Here's how the part is built. I have some questions about the finished solid (model axes, mm). A direction names the side the tool comes from. Coordinates: 2 decimals unless noted, no trailing zeros. Order: outer loops, then holes, each group sorted by start corner. A loop starts at its lowest first (then second) coordinate and runs counter-clockwise, first axis right, second up. Notation, with made-up numbers: M 62.5,10.5 L 77.5,10.5 A36 ccw 77.5,46.5 Z; hole C 52.25,15.5 d4. An arc over 180 degrees is marked long. One line per question, with ' | ' between items. Start each with the question number.
```python
from build123d import *

# Parameters (mm, degrees)
MAIN_5_W                = 20
MAIN_5_H                = 12.7
BOSS_EXTRUDE2_DEPTH     = 6.35
CUT_EXTRUDE1_DEPTH      = 300.179502974
CUT_EXTRUDE1_DEPTH_BACK = 300.179502974
SKETCH1_W               = 12.7
SKETCH1_H               = 20
M8_CLEARANCE_HOLE2_D    = 9
CUT_EXTRUDE2_DEPTH      = 300.179502974
CUT_EXTRUDE2_DEPTH_BACK = 300.179502974
SKETCH6_R               = 4
SKETCH6_R_2             = 3.175
SKETCH6_R_3             = 1.25
CUT_EXTRUDE3_DEPTH      = 300.179502974
CUT_EXTRUDE3_DEPTH_BACK = 300.179502974
SKETCH7_R               = 25
F_6_0MM_DOWEL_HOLE2_D   = 6


with BuildPart() as part:
    # MAIN<5> → Boss-Extrude2 (new, symmetric)
    with BuildSketch(Plane(origin=(0, 0, 0), x_dir=(1, 0, 0), z_dir=(0, 1, 0))):
        Polygon((-271.75, 92.5), (-271.75, 79.8), (-284.45, 79.8), (-284.45, 59.8), (-271.75, 59.8), (-271.75, 4), (-266.45, 4), (-266.45, 6.5), (-259.45, 6.5), (-259.45, 4), (-256.45, 4), (-256.45, -4), (-259.45, -4), (-259.45, -6.5), (-266.45, -6.5), (-266.45, -4), (-271.75, -4), (-271.75, -59.8), (-284.45, -59.8), (-284.45, -79.8), (-271.75, -79.8), (-271.75, -92.5), (271.75, -92.5), (271.75, -79.8), (284.45, -79.8), (284.45, -59.8), (271.75, -59.8), (271.75, -4), (266.45, -4), (266.45, -6.5), (259.45, -6.5), (259.45, -4), (256.45, -4), (256.45, 4), (259.45, 4), (259.45, 6.5), (266.45, 6.5), (266.45, 4), (271.75, 4), (271.75, 59.8), (284.45, 59.8), (284.45, 79.8), (271.75, 79.8), (271.75, 92.5), align=None)
        with Locations((-157.7, 0)):
            Rectangle(MAIN_5_W, MAIN_5_H, mode=Mode.SUBTRACT)
        with Locations((-107.7, 0)):
            Rectangle(MAIN_5_W, MAIN_5_H, mode=Mode.SUBTRACT)
        with Locations((107.7, 0)):
            Rectangle(MAIN_5_W, MAIN_5_H, mode=Mode.SUBTRACT)
        with Locations((157.7, 0)):
            Rectangle(MAIN_5_W, MAIN_5_H, mode=Mode.SUBTRACT)
    extrude(amount=BOSS_EXTRUDE2_DEPTH, both=True)

    # Sketch1 → Cut-Extrude1 (cut, two sides: drawn at the far end of the back side and taken through both)
    with BuildSketch(Plane(origin=(0, 0, 0), x_dir=(1, 0, 0), z_dir=(0, 1, 0)).offset(-CUT_EXTRUDE1_DEPTH_BACK)):
        with Locations((0, 69.8)):
            Rectangle(SKETCH1_W, SKETCH1_H)
        with Locations((0, -69.8)):
            Rectangle(SKETCH1_W, SKETCH1_H)
    extrude(amount=CUT_EXTRUDE1_DEPTH + CUT_EXTRUDE1_DEPTH_BACK, mode=Mode.SUBTRACT)

    # M8 Clearance Hole2 (through all)
    with Locations(Plane(origin=(0, 6.35, 0), x_dir=(1, 0, 0), z_dir=(0, 1, 0))):
        with Locations((-132.7, 0), (132.7, 0), (0, 0)):
            Hole(M8_CLEARANCE_HOLE2_D / 2)

    # Sketch6 → Cut-Extrude2 (cut, two sides: drawn at the far end of the back side and taken through both)
    with BuildSketch(Plane(origin=(0, 0, 0), x_dir=(1, 0, 0), z_dir=(0, 1, 0)).offset(-CUT_EXTRUDE2_DEPTH_BACK)):
        with Locations(Location((-199.05, -61.85, 0), (0, 0, 270))):
            Circle(SKETCH6_R)
        with Locations(Location((-199.05, -70.85, 0), (0, 0, 270))):
            Circle(SKETCH6_R_2)
        with Locations(Location((-205.05, -66.35, 0), (0, 0, 270))):
            Circle(SKETCH6_R_3)
        with Locations(Location((-193.05, -66.35, 0), (0, 0, 270))):
            Circle(SKETCH6_R_3)
        with Locations(Location((-66.35, -70.85, 0), (0, 0, 270))):
            Circle(SKETCH6_R_2)
        with Locations(Location((-66.35, -61.85, 0), (0, 0, 270))):
            Circle(SKETCH6_R)
        with Locations(Location((-72.35, -66.35, 0), (0, 0, 270))):
            Circle(SKETCH6_R_3)
        with Locations(Location((-60.35, -66.35, 0), (0, 0, 270))):
            Circle(SKETCH6_R_3)
        with Locations(Location((66.35, -70.85, 0), (0, 0, 270))):
            Circle(SKETCH6_R_2)
        with Locations(Location((66.35, -61.85, 0), (0, 0, 270))):
            Circle(SKETCH6_R)
        with Locations(Location((60.35, -66.35, 0), (0, 0, 270))):
            Circle(SKETCH6_R_3)
        with Locations(Location((72.35, -66.35, 0), (0, 0, 270))):
            Circle(SKETCH6_R_3)
        with Locations(Location((199.05, -70.85, 0), (0, 0, 270))):
            Circle(SKETCH6_R_2)
        with Locations(Location((199.05, -61.85, 0), (0, 0, 270))):
            Circle(SKETCH6_R)
        with Locations(Location((193.05, -66.35, 0), (0, 0, 270))):
            Circle(SKETCH6_R_3)
        with Locations(Location((205.05, -66.35, 0), (0, 0, 270))):
            Circle(SKETCH6_R_3)
        with Locations(Location((205.05, 66.35, 0), (0, 0, 90))):
            Circle(SKETCH6_R_3)
        with Locations(Location((193.05, 66.35, 0), (0, 0, 90))):
            Circle(SKETCH6_R_3)
        with Locations(Location((199.05, 61.85, 0), (0, 0, 90))):
            Circle(SKETCH6_R)
        with Locations(Location((199.05, 70.85, 0), (0, 0, 90))):
            Circle(SKETCH6_R_2)
        with Locations(Location((72.35, 66.35, 0), (0, 0, 90))):
            Circle(SKETCH6_R_3)
        with Locations(Location((60.35, 66.35, 0), (0, 0, 90))):
            Circle(SKETCH6_R_3)
        with Locations(Location((66.35, 61.85, 0), (0, 0, 90))):
            Circle(SKETCH6_R)
        with Locations(Location((66.35, 70.85, 0), (0, 0, 90))):
            Circle(SKETCH6_R_2)
        with Locations(Location((-60.35, 66.35, 0), (0, 0, 90))):
            Circle(SKETCH6_R_3)
        with Locations(Location((-72.35, 66.35, 0), (0, 0, 90))):
            Circle(SKETCH6_R_3)
        with Locations(Location((-66.35, 61.85, 0), (0, 0, 90))):
            Circle(SKETCH6_R)
        with Locations(Location((-66.35, 70.85, 0), (0, 0, 90))):
            Circle(SKETCH6_R_2)
        with Locations(Location((-193.05, 66.35, 0), (0, 0, 90))):
            Circle(SKETCH6_R_3)
        with Locations(Location((-205.05, 66.35, 0), (0, 0, 90))):
            Circle(SKETCH6_R_3)
        with Locations(Location((-199.05, 70.85, 0), (0, 0, 90))):
            Circle(SKETCH6_R_2)
        with Locations(Location((-199.05, 61.85, 0), (0, 0, 90))):
            Circle(SKETCH6_R)
    extrude(amount=CUT_EXTRUDE2_DEPTH + CUT_EXTRUDE2_DEPTH_BACK, mode=Mode.SUBTRACT)

    # Sketch7 → Cut-Extrude3 (cut, two sides: drawn at the far end of the back side and taken through both)
    with BuildSketch(Plane(origin=(0, 0, 0), x_dir=(1, 0, 0), z_dir=(0, 1, 0)).offset(-CUT_EXTRUDE3_DEPTH_BACK)):
        with Locations(Location((-132.7, -46.25, 0), (0, 0, 270))):
            Circle(SKETCH7_R)
        with Locations(Location((132.7, -46.25, 0), (0, 0, 270))):
            Circle(SKETCH7_R)
        with Locations(Location((132.7, 46.25, 0), (0, 0, 90))):
            Circle(SKETCH7_R)
        with Locations(Location((-132.7, 46.25, 0), (0, 0, 90))):
            Circle(SKETCH7_R)
        with Locations(Location((-219.725, 0, 0), (0, 0, 270))):
            Circle(SKETCH7_R)
        with Locations(Location((-52.025, 0, 0), (0, 0, 270))):
            Circle(SKETCH7_R)
        with Locations(Location((52.025, 0, 0), (0, 0, 90))):
            Circle(SKETCH7_R)
        with Locations(Location((219.725, 0, 0), (0, 0, 90))):
            Circle(SKETCH7_R)
    extrude(amount=CUT_EXTRUDE3_DEPTH + CUT_EXTRUDE3_DEPTH_BACK, mode=Mode.SUBTRACT)

    # Ø6.0mm Dowel Hole2 (through all)
    with Locations(Plane(origin=(0, 6.35, 0), x_dir=(1, 0, 0), z_dir=(0, 1, 0))):
        with Locations((-256.45, -86.5), (-183.178571429, -86.5), (-109.907142857, -86.5), (-36.635714286, -86.5), (36.635714286, -86.5), (109.907142857, -86.5), (183.178571429, -86.5), (256.45, -86.5), (256.45, 86.5), (183.178571429, 86.5), (109.907142857, 86.5), (36.635714286, 86.5), (-36.635714286, 86.5), (-109.907142857, 86.5), (-183.178571429, 86.5), (-256.45, 86.5)):
            Hole(F_6_0MM_DOWEL_HOLE2_D / 2)


solid = part.part
```
1. Will these pins go through, and if not, where does the flat tip stop? pin 1 (2 mm diameter, centred on y = 1, z = -52.5, fed in from -X); pin 2 (5 mm diameter, centred on x = -66.35, z = 61.85, fed in from +Y); pin 3 (4 mm diameter, centred on x = -279, y = 1.5, fed in from +Z); pin 4 (4 mm diameter, centred on y = 2.5, z = 1.5, fed in from -X).
2. We'd pull the mould along X, two halves only. Please class faces 1 (the face through (-4, 6.35, -22)), 2 (the face through (244.13, -0.09, 5.42)), 3 (the face through (271.75, 0, -86)): released by +X, released by -X, zero draft, split by the parting line, or undercut.
3. Imagine slicing it at A-A (z = -46.25). List the corners of the cut face in (x, y) for me, then the cut area to 3 significant figures.
4. Imagine slicing it at B-B (x = -46). List the corners of the cut face in (y, z) for me, then the cut area to 3 significant figures.
5. I need wall thicknesses on line 1 (Z direction, x = -217.5, y = 4.75); line 2 (Z direction, x = -199.05, y = 2) (3 decimals); line 3 (Z direction, x = 150.5, y = -1.75). Which ranges of each line are inside material? Lowest first, please.
6. Imagine slicing it at C-C (z = 16). List the corners of the cut face in (x, y) for me.
7. Which directions (+Z, -Z, +X, -X, +Y, -Y) give clear straight access to the entire face, cutting with the end or side of a thin tool? Please do faces 4 (the face through (278, 0, 59.8)), 5 (the face through (97.7, 0, 0)), 6 (the face through (-271.75, 0, -86)).
8. Imagine slicing it at D-D (y = 3.75). Count the separate pieces of the cut face and the enclosed holes in it, then the cut area to 3 significant figures.
Entries:
1) pin 1: x = -271.75 | pin 2: through | pin 3: z = 79.8 | pin 4: x = -256.45
2) face 1: zero draft | face 2: undercut | face 3: released by +X
3) outline: M -271.75,-6.35 L -157.7,-6.35 L -157.7,6.35 L -271.75,6.35 Z; M -107.7,-6.35 L 107.7,-6.35 L 107.7,6.35 L -107.7,6.35 Z; M 157.7,-6.35 L 271.75,-6.35 L 271.75,6.35 L 157.7,6.35 Z | area: 5,630 mm²
4) outline: M -6.35,-92.5 L 6.35,-92.5 L 6.35,-24.26 L -6.35,-24.26 Z; M -6.35,24.26 L 6.35,24.26 L 6.35,92.5 L -6.35,92.5 Z | area: 1,730 mm²
5) line 1: -92.5 to -24.9, 24.9 to 92.5 | line 2: -92.5 to -74.025, -67.675 to -65.85, -57.85 to -14.055, 14.055 to 57.85, 65.85 to 67.675, 74.025 to 92.5 | line 3: -92.5 to -63.8, -28.7 to -6.35, 6.35 to 28.7, 63.8 to 92.5
6) outline: M -271.75,-6.35 L -238.93,-6.35 L -238.93,6.35 L -271.75,6.35 Z; M -200.52,-6.35 L -71.23,-6.35 L -71.23,6.35 L -200.52,6.35 Z; M -32.82,-6.35 L 32.82,-6.35 L 32.82,6.35 L -32.82,6.35 Z; M 71.23,-6.35 L 200.52,-6.35 L 200.52,6.35 L 71.23,6.35 Z; M 238.93,-6.35 L 271.75,-6.35 L 271.75,6.35 L 238.93,6.35 Z
7) face 4: +X, +Y, -Y | face 5: +Y, -Y | face 6: -Z, -X, +Y, -Y
8) separate pieces: 1 | enclosed holes: 65 | area: 82,600 mm²
